Geometry: see drawing. Coordinates: mm, zero at the bounding-box minimum. A direction names the side the tool comes from. Coordinates: 2 decimals unless noted, no trailing zeros. Write each loop counter-clockwise with the first axis right and the second up, starting at its lowest first coordinate (ties: lowest second). Pieces come first, ordered by that corner, then holes.
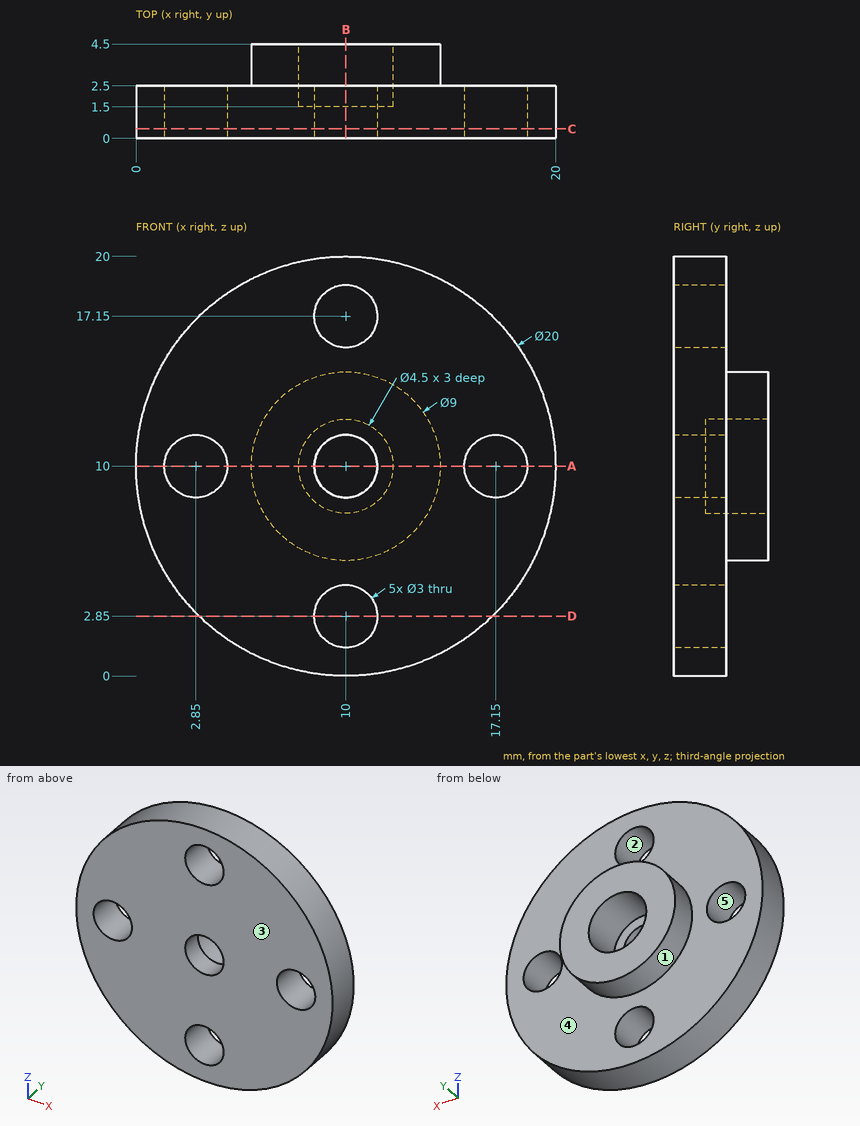
Item 1: Section C-C, the plane y = 0.45. Output: boundary loops of the cut face in (x, z), plus the area to 3 significant figures.
Derived:
outline: circle Ø20 at (10, 10); hole circle Ø3 at (2.85, 10); hole circle Ø3 at (10, 2.85); hole circle Ø3 at (10, 10); hole circle Ø3 at (10, 17.15); hole circle Ø3 at (17.15, 10)
area: 279 mm2
Item 2: Pin query (flat end, axial travel): pin 1 (2 mm diameter, centred on x = 7.5, z = 17, fed in from +Y); pin 2 (1.3 mm diameter, centred on x = 9, z = 11, fed in from +Y); pin 3 (1 mm diameter, centred on x = 13.5, y = 2, fed in from +Z). Return the tip coordinate at first contact, or that it passes through.
Derived:
pin 1: stops at y = 2.5
pin 2: stops at y = 1.5
pin 3: stops at z = 19.54
Item 3: Section A-A, the plane z = 10. Output: boundary loops of the cut face in (x, y), plus the area to 3 significant figures.
Derived:
outline: (0, 0) - (1.35, 0) - (1.35, 2.5) - (0, 2.5) - close; (4.35, 0) - (8.5, 0) - (8.5, 1.5) - (7.75, 1.5) - (7.75, 4.5) - (5.5, 4.5) - (5.5, 2.5) - (4.35, 2.5) - close; (11.5, 0) - (15.65, 0) - (15.65, 2.5) - (14.5, 2.5) - (14.5, 4.5) - (12.25, 4.5) - (12.25, 1.5) - (11.5, 1.5) - close; (18.65, 0) - (20, 0) - (20, 2.5) - (18.65, 2.5) - close
area: 35.0 mm2
Item 4: Section B-B, the plane x = 10. Output: boundary loops of the cut face in (y, z).
Derived:
outline: (0, 0) - (2.5, 0) - (2.5, 1.35) - (0, 1.35) - close; (0, 4.35) - (2.5, 4.35) - (2.5, 5.5) - (4.5, 5.5) - (4.5, 7.75) - (1.5, 7.75) - (1.5, 8.5) - (0, 8.5) - close; (0, 11.5) - (1.5, 11.5) - (1.5, 12.25) - (4.5, 12.25) - (4.5, 14.5) - (2.5, 14.5) - (2.5, 15.65) - (0, 15.65) - close; (0, 18.65) - (2.5, 18.65) - (2.5, 20) - (0, 20) - close
Item 5: Set-up query: the marked faces 4 and 5. Return all of +Z, -Z, +X, -X, +Y, -Y with unobstructed straight access to the full face (end or side cutting, diameter ignored); none if empty.
Derived:
face 4: +Y
face 5: +Y, -Y
Item 6: Pull-direction query (X, two-part tool) for the marked faces 1, 2 and 3; classes: released by +X, released by -X, zero draft, split by the parting line, or undercut.
Derived:
face 1: split by the parting line
face 2: undercut
face 3: zero draft
Item 7: Section D-D, the plane z = 2.85. Output: boundary loops of the cut face in (x, y), plus the area to 3 significant figures.
Derived:
outline: (3.01, 0) - (8.5, 0) - (8.5, 2.5) - (3.01, 2.5) - close; (11.5, 0) - (16.99, 0) - (16.99, 2.5) - (11.5, 2.5) - close
area: 27.5 mm2
Item 8: Material intervals for probe 1 along X at (y, z) = (1, 10); probe 2 along Z at (x, y) = (12, 2.1); probe 3 along Y at (x, z) = (13.5, 13.5), sorted ascending.
Derived:
probe 1: x = 0 to 1.35, 4.35 to 8.5, 11.5 to 15.65, 18.65 to 20
probe 2: z = 0.2 to 8.97, 11.03 to 19.8
probe 3: y = 0 to 2.5
